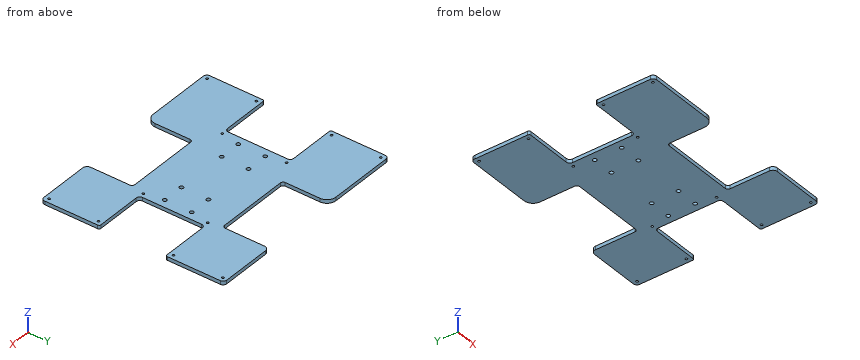
from build123d import *

# Parameters (mm, degrees)
SKETCH1_R                = 1.5
SKETCH1_R_2              = 1
BOSS_EXTRUDE1_DEPTH      = 4
M4_CLEARANCE_HOLE1_D     = 4.3
M4_CLEARANCE_HOLE1_DEPTH = 6
M4_CLEARANCE_HOLE1_TIP   = 1.291850331
M3_TAPPED_HOLE1_D        = 2.5
M3_TAPPED_HOLE1_DEPTH    = 7.5
M3_TAPPED_HOLE1_TIP      = 0.751075774


with BuildPart() as part:
    # Sketch1 → Boss-Extrude1 (new body)
    with BuildSketch(Plane.XY):
        with BuildLine():
            Line((-119, 97.846596312), (-119, 38.84934343))
            ThreePointArc((-119, 38.84934343), (-118.414213562, 37.435129868), (-117, 36.84934343))
            Line((-117, 36.84934343), (-65.999162166, 36.84934343))
            ThreePointArc((-65.999162166, 36.84934343), (-63.170735042, 35.677770555), (-61.999162166, 32.84934343))
            Line((-61.999162166, 32.84934343), (-61.999162166, -32.84934343))
            ThreePointArc((-61.999162166, -32.84934343), (-63.170735042, -35.677770555), (-65.999162166, -36.84934343))
            Line((-65.999162166, -36.84934343), (-117, -36.84934343))
            ThreePointArc((-117, -36.84934343), (-118.414213562, -37.435129868), (-119, -38.84934343))
            Line((-119, -38.84934343), (-119, -97.846596312))
            ThreePointArc((-119, -97.846596312), (-117.828427125, -100.675023437), (-115, -101.846596312))
            Line((-115, -101.846596312), (-42.690502092, -101.846596312))
            ThreePointArc((-42.690502092, -101.846596312), (-35.61943428, -98.917664124), (-32.690502092, -91.846596312))
            Line((-32.690502092, -91.846596312), (-32.690502092, -53.007425707))
            ThreePointArc((-32.690502092, -53.007425707), (-31.811822435, -50.886105364), (-29.690502092, -50.007425707))
            Line((-29.690502092, -50.007425707), (51.077147655, -50.007425707))
            ThreePointArc((51.077147655, -50.007425707), (53.198467999, -50.886105364), (54.077147655, -53.007425707))
            Line((54.077147655, -53.007425707), (54.077147655, -96.846596312))
            ThreePointArc((54.077147655, -96.846596312), (55.541613749, -100.382130218), (59.077147655, -101.846596312))
            Line((59.077147655, -101.846596312), (115, -101.846596312))
            ThreePointArc((115, -101.846596312), (117.828427125, -100.675023437), (119, -97.846596312))
            Line((119, -97.846596312), (119, -38.84934343))
            ThreePointArc((119, -38.84934343), (118.414213562, -37.435129868), (117, -36.84934343))
            Line((117, -36.84934343), (65.999162166, -36.84934343))
            ThreePointArc((65.999162166, -36.84934343), (63.170735042, -35.677770555), (61.999162166, -32.84934343))
            Line((61.999162166, -32.84934343), (61.999162166, 32.84934343))
            ThreePointArc((61.999162166, 32.84934343), (63.170735042, 35.677770555), (65.999162166, 36.84934343))
            Line((65.999162166, 36.84934343), (117, 36.84934343))
            ThreePointArc((117, 36.84934343), (118.414213562, 37.435129868), (119, 38.84934343))
            Line((119, 38.84934343), (119, 97.846596312))
            ThreePointArc((119, 97.846596312), (117.828427125, 100.675023437), (115, 101.846596312))
            Line((115, 101.846596312), (59.077147655, 101.846596312))
            ThreePointArc((59.077147655, 101.846596312), (55.541613749, 100.382130218), (54.077147655, 96.846596312))
            Line((54.077147655, 96.846596312), (54.077147655, 53.007425707))
            ThreePointArc((54.077147655, 53.007425707), (53.198467999, 50.886105364), (51.077147655, 50.007425707))
            Line((51.077147655, 50.007425707), (29.690502092, 50.007425707))
            Line((29.690502092, 50.007425707), (-29.690502092, 50.007425707))
            ThreePointArc((-29.690502092, 50.007425707), (-31.811822435, 50.886105364), (-32.690502092, 53.007425707))
            Line((-32.690502092, 53.007425707), (-32.690502092, 91.846596312))
            ThreePointArc((-32.690502092, 91.846596312), (-35.61943428, 98.917664124), (-42.690502092, 101.846596312))
            Line((-42.690502092, 101.846596312), (-115, 101.846596312))
            ThreePointArc((-115, 101.846596312), (-117.828427125, 100.675023437), (-119, 97.846596312))
        make_face()
        with Locations(Location((29, 15, 0), (0, 0, 180))):
            Circle(SKETCH1_R, mode=Mode.SUBTRACT)
        with Locations(Location((53, 15, 0), (0, 0, 180))):
            Circle(SKETCH1_R, mode=Mode.SUBTRACT)
        with Locations(Location((53, -15, 0), (0, 0, 180))):
            Circle(SKETCH1_R, mode=Mode.SUBTRACT)
        with Locations(Location((29, -15, 0), (0, 0, 180))):
            Circle(SKETCH1_R, mode=Mode.SUBTRACT)
        with Locations((-114, 41.84934343)):
            Circle(SKETCH1_R_2, mode=Mode.SUBTRACT)
        with Locations((-56.999162166, 35.84934343)):
            Circle(SKETCH1_R_2, mode=Mode.SUBTRACT)
        with Locations((-114, 96.846596312)):
            Circle(SKETCH1_R_2, mode=Mode.SUBTRACT)
        with Locations(Location((114, 96.846596312, 0), (0, 0, 180))):
            Circle(SKETCH1_R_2, mode=Mode.SUBTRACT)
        with Locations(Location((56.999162166, 35.84934343, 0), (0, 0, 180))):
            Circle(SKETCH1_R_2, mode=Mode.SUBTRACT)
        with Locations((-29, -15)):
            Circle(SKETCH1_R, mode=Mode.SUBTRACT)
        with Locations((-53, -15)):
            Circle(SKETCH1_R, mode=Mode.SUBTRACT)
        with Locations((-53, 15)):
            Circle(SKETCH1_R, mode=Mode.SUBTRACT)
        with Locations((-29, 15)):
            Circle(SKETCH1_R, mode=Mode.SUBTRACT)
        with Locations(Location((114, 41.84934343, 0), (0, 0, 180))):
            Circle(SKETCH1_R_2, mode=Mode.SUBTRACT)
        with Locations((114, -96.846596312)):
            Circle(SKETCH1_R_2, mode=Mode.SUBTRACT)
        with Locations((114, -41.84934343)):
            Circle(SKETCH1_R_2, mode=Mode.SUBTRACT)
        with Locations((56.999162166, -35.84934343)):
            Circle(SKETCH1_R_2, mode=Mode.SUBTRACT)
        with Locations(Location((-56.999162166, -35.84934343, 0), (0, 0, 180))):
            Circle(SKETCH1_R_2, mode=Mode.SUBTRACT)
        with Locations(Location((-114, -96.846596312, 0), (0, 0, 180))):
            Circle(SKETCH1_R_2, mode=Mode.SUBTRACT)
        with Locations(Location((-114, -41.84934343, 0), (0, 0, 180))):
            Circle(SKETCH1_R_2, mode=Mode.SUBTRACT)
    extrude(amount=BOSS_EXTRUDE1_DEPTH)

    # M4 Clearance Hole1
    with Locations(Plane(origin=(-53, 15, 4), x_dir=(1, 0, 0), z_dir=(0, 0, 1))):
        with Locations((0, 0), (24, 0), (0, -30), (24, -30), (82, -30), (106, -30), (106, 0), (82, 0)):
            Hole(M4_CLEARANCE_HOLE1_D / 2, depth=M4_CLEARANCE_HOLE1_DEPTH)
            with Locations((0, 0, -(M4_CLEARANCE_HOLE1_DEPTH + M4_CLEARANCE_HOLE1_TIP / 2))):  # 118° drill point
                Cone(0, M4_CLEARANCE_HOLE1_D / 2, M4_CLEARANCE_HOLE1_TIP, mode=Mode.SUBTRACT)

    # M3 Tapped Hole1
    with Locations(Plane(origin=(-114, -96.846596312, 4), x_dir=(1, 0, 0), z_dir=(0, 0, 1))):
        with Locations((0, 0), (228, 0), (228, 54.997252882), (170.999162166, 60.997252882), (57.000837834, 60.997252882), (0, 54.997252882), (0, 138.695939742), (57.000837834, 132.695939742), (0, 193.693192624), (170.999162166, 132.695939742), (228, 138.695939742), (228, 193.693192624)):
            Hole(M3_TAPPED_HOLE1_D / 2, depth=M3_TAPPED_HOLE1_DEPTH)
            with Locations((0, 0, -(M3_TAPPED_HOLE1_DEPTH + M3_TAPPED_HOLE1_TIP / 2))):  # 118° drill point
                Cone(0, M3_TAPPED_HOLE1_D / 2, M3_TAPPED_HOLE1_TIP, mode=Mode.SUBTRACT)


solid = part.part
Can you work these out from the model? Positions are in its coordinate system, mm. Give positions to 0.01 mm unless a question says otherwise; leave off trailing zeros. Loops run counter-clockwise (first coordinate to the right, second up) from the corner with the lowest first, then second, coordinate; pieces in that order, holes last. Notation, with made-up numbers: M 46.25,-24.75 L 81.25,-24.75 A22 ccw 81.25,0.25 Z; hole C -31,42.25 d4. An arc over 180 degrees is marked long. One line per item, written item: value. Start each with the question number.
1) I'm going to push a flat-ended pin straight in: pin 1 (2 mm diameter, centred on y = 16, z = 2, fed in from -X). Where does the tip first touch, or does it pass through?
2) If we section it at A-A, the plane x = -99.5: Write out the boundary of the cut face in (y, z).
3) If I drill on line 1 (Y direction, x = 114, z = 0.85); line 2 (X direction, y = -89.5, z = 0.6); line 3 (Y direction, x = -29, z = 1.85), over which ranges is the centre line in solid material (lowest first)? Write a range as [from, to].
4) If we section it at D-D, the plane z = 3: Give the number of separate pieces and of enclosed holes in the cut face, and give its area (3 significant figures).
5) If we section it at C-C, the plane x = 44: Write out the boundary of the cut face in (y, z).
6) If we section it at B-B, the plane y = 80: Write out the boundary of the cut face in (x, z).
Completed:
1. pin 1: stops at x = -62
2. outline: M -101.85,0 L -36.85,0 L -36.85,4 L -101.85,4 Z; M 36.85,0 L 101.85,0 L 101.85,4 L 36.85,4 Z
3. line 1: y = [-101.85, -98.1], [-95.6, -43.1], [-40.6, -36.85], [36.85, 40.6], [43.1, 95.6], [98.1, 101.85]
3. line 2: x = [-119, -32.69], [54.08, 119]
3. line 3: y = [-50.01, -17.15], [-12.85, 12.85], [17.15, 50.01]
4. separate pieces: 1
4. enclosed holes: 20
4. area: 30,900 mm^2
5. outline: M -50.01,0 L 50.01,0 L 50.01,4 L -50.01,4 Z
6. outline: M -119,0 L -32.69,0 L -32.69,4 L -119,4 Z; M 54.08,0 L 119,0 L 119,4 L 54.08,4 Z
